```python
from build123d import *

# Parameters (mm, degrees)
BASENUT_START = -5
BASENUTSKE_W  = 17
BASENUTSKE_H  = 17
BASENUTSKE_R  = 4.25
BASENUT_DEPTH = 5


with BuildPart() as part:
    # BaseNutSke → BaseNut (new body)
    with BuildSketch(Plane.XY.offset(BASENUT_START)):
        Rectangle(BASENUTSKE_W, BASENUTSKE_H)
        Circle(BASENUTSKE_R, mode=Mode.SUBTRACT)
    extrude(amount=BASENUT_DEPTH)

    # EndChamferSketch → EndChamfer (revolve, cut)
    with BuildSketch(Plane(origin=(0, 0, 0), x_dir=(0, 0, -1), z_dir=(1, 0, 0)), mode=Mode.PRIVATE) as endchamfer_sk:
        Polygon((4.991, 5), (4.413328781, 4.175), (5.001, 4.175), (5.001, 5), align=None)
        Polygon((-0.002, 5), (0.008, 5), (0.585671219, 4.175), (-0.002, 4.175), align=None)
    revolve(endchamfer_sk.sketch.rotate(Axis((0, 0, -25.037505729), (0, 0, -1)), 90), axis=Axis((0, 0, -25.037505729), (0, 0, -1)), mode=Mode.SUBTRACT)


solid = part.part
```
Input: part model. Units: mm. Frame: model coordinates. Round coordinates to 2 decimals unless told otherwise and drop trailing zeros. Loops run counter-clockwise (first coordinate to the right, second up) from the corner with the lowest first, then second, coordinate; pieces in that order, holes last. Notation, with made-up numbers: (24, 50.25) -> (58, 50.25) arc R21 cw to (58, 61.25) -> close; hole circle Ø3 at (51.25, 0). An arc over 180 degrees is marked (long way). Use one line per item in the form item = value. Start each with the question number.
Item 1: Section query C-C on z = -1.1. Return the cut outline in (x, y).
Item 2: Mould query, pull axis Y, two halves, no side actions, for faces 1 (the face through (2.285, 3.584, -2.527)), 2 (the face through (0, -8.5, -3)), 3 (the face through (0, 8.5, -3)), 4 (the face through (4, 4, 0)). Classes: pulls with the +Y half, pulls with the -Y half, needs draft (parallel to the pull), parting line crosses it, or undercut.
Item 3: Material intervals for L1, parallel to Y at x = 0, z = -2.45; L2, parallel to Z at x = -5, y = 0; L3, parallel to Y at x = -2.25, z = -3.7, sorted ascending. Write a range as from..to.
Ans:
q1.outline = (-8.5, -8.5) -> (8.5, -8.5) -> (8.5, 8.5) -> (-8.5, 8.5) -> close; hole circle Ø8.5 at (0, 0)
q2.face_1 = undercut
q2.face_2 = pulls with the -Y half
q2.face_3 = pulls with the +Y half
q2.face_4 = needs draft
q3.L1 = -8.5..-4.25, 4.25..8.5
q3.L2 = -4.99..-0.01
q3.L3 = -8.5..-3.61, 3.61..8.5
